Source: CAD feature listing. Evaluate the final solid. Frame: model axes, mm. A direction names the side the tool comes from. Give positions to 0.01 mm unless a question says otherwise; leave off trailing zeros. Loops run counter-clockwise (first coordinate to the right, second up) from the corner with the lowest first, then second, coordinate; pieces in that order, holes last.
from build123d import *

# Parameters (mm, degrees)
BOSS_EXTRUDE1_DEPTH            = 62
CONVERT_SOLID1_DEPTH           = 62
CONVERT_SOLID1_2_DEPTH         = 62
CUT_EXTRUDE2_DEPTH             = 79.552402891
SKETCH9_W                      = 18.8
SKETCH9_H                      = 20
CUT_EXTRUDE3_DEPTH             = 79.552402891
BOSS_EXTRUDE3_DEPTH            = 1.2
BOSS_EXTRUDE4_DEPTH            = 20
CUT_EXTRUDE4_DEPTH             = 20.58
CUT_EXTRUDE4_DIRECTION_2_REACH = 81.822
CHAMFER4_SIZE                  = 4
CHAMFER1_SIZE                  = 1.5
SKETCH7_R                      = 2.7686
CUT_EXTRUDE1_DEPTH             = 1.2


# Read off the part's stored shape, not the designer's step: Convert-Solid1
with BuildPart() as part:
    # Sketch2 → Boss-Extrude1 (new body)
    with BuildSketch(Plane(origin=(0, 0, 0), x_dir=(1, 0, 0), z_dir=(0, 1, 0))):
        Polygon((10, 0), (3, 0), (-3.915434451, 19), (-43.8, 19), (-43.8, 40), (10, 40), align=None)
    extrude(amount=BOSS_EXTRUDE1_DEPTH)

    # Convert-Solid1 outline → Convert-Solid1 (cut)
    with BuildSketch(Plane(origin=(0, 0, 0), x_dir=(1, 0, 0), z_dir=(0, 1, 0))):
        with BuildLine():
            ThreePointArc((4.680498092, 0), (3.303914645, 0.434035094), (2.425235802, 1.579151656))
            Line((2.425235802, 1.579151656), (3, 0))
            Line((3, 0), (4.680498092, 0))
        make_face()
        with BuildLine():
            Line((-43.8, 40), (-43.8, 20.2))
            Line((-43.8, 20.2), (-4.755683497, 20.2))
            ThreePointArc((-4.755683497, 20.2), (-3.37910005, 19.765964906), (-2.500421207, 18.620848344))
            Line((-2.500421207, 18.620848344), (3.552866947, 1.989575828))
            ThreePointArc((3.552866947, 1.989575828), (3.992206368, 1.417017547), (4.680498092, 1.2))
            Line((4.680498092, 1.2), (10, 1.2))
            Line((10, 1.2), (10, 40))
            Line((10, 40), (-43.8, 40))
        make_face()
    extrude(amount=CONVERT_SOLID1_DEPTH, mode=Mode.SUBTRACT)

    # Convert-Solid1 2 outline → Convert-Solid1 2 (add)
    with BuildSketch(Plane(origin=(0, 0, 0), x_dir=(1, 0, 0), z_dir=(0, 1, 0))):
        with BuildLine():
            ThreePointArc((-4.755683497, 19), (-4.067391773, 18.782982453), (-3.628052352, 18.210424172))
            Line((-3.628052352, 18.210424172), (-3.915434451, 19))
            Line((-3.915434451, 19), (-4.755683497, 19))
        make_face()
    extrude(amount=CONVERT_SOLID1_2_DEPTH)

    # Sketch8 → Cut-Extrude2 (cut, through all)
    with BuildSketch(Plane.XY):
        Polygon((-8.8, 35), (-10.3748, 34.347696482), (-10.3748, -34.347696482), (-8.8, -35), align=None)
        Polygon((-8.8, 35.5), (-10.3748, 36.152303518), (-10.3748, 75), (-8.8, 75), align=None)
        Polygon((-10.3748, -36.152303518), (-10.3748, -75), (-8.8, -75), (-8.8, -35.5), align=None)
    extrude(amount=-CUT_EXTRUDE2_DEPTH, mode=Mode.SUBTRACT)

    # Sketch9 → Cut-Extrude3 (cut, through all)
    with BuildSketch(Plane.XY):
        with Locations((0.6, 52)):
            Rectangle(SKETCH9_W, SKETCH9_H)
    extrude(amount=-CUT_EXTRUDE3_DEPTH, mode=Mode.SUBTRACT)

    # Sketch11 → Boss-Extrude3 (add)
    with BuildSketch(Plane.XY):
        Polygon((-3.1496, 43.5748), (4.680498092, 43.5748), (4.680498092, 42), (10, 42), (10, 62), (-10, 62), (-10, 50.4252), align=None)
    extrude(amount=-BOSS_EXTRUDE3_DEPTH)

    # Sketch12 → Boss-Extrude4 (add)
    with BuildSketch(Plane(origin=(0, 42, 0), x_dir=(1, 0, 0), z_dir=(0, 1, 0))):
        with BuildLine():
            Line((-3.628052352, 18.210424172), (0.305179296, 7.403959033))
            Line((0.305179296, 7.403959033), (1.432810441, 7.814383205))
            Line((1.432810441, 7.814383205), (-2.500421207, 18.620848344))
            ThreePointArc((-2.500421207, 18.620848344), (-3.37910005, 19.765964906), (-4.755683497, 20.2))
            Line((-4.755683497, 20.2), (-8.8, 20.2))
            Line((-8.8, 20.2), (-8.8, 19))
            Line((-8.8, 19), (-4.755683497, 19))
            ThreePointArc((-4.755683497, 19), (-4.067391773, 18.782982453), (-3.628052352, 18.210424172))
        make_face()
    extrude(amount=BOSS_EXTRUDE4_DEPTH)

    # Sketch13 → Cut-Extrude4 (cut)
    with BuildSketch(Plane(origin=(2.649066665, 0, -0.964181415), x_dir=(0.34202014332566943, 0, 0.9396926207859082), z_dir=(-0.9396926207859082, 0, 0.34202014332566943))):
        Polygon((-6.853068201, 42), (-11.853068201, 47), (-26.853068201, 47), (-26.853068201, 62), (-6.853068201, 62), align=None)
    extrude(amount=-CUT_EXTRUDE4_DEPTH, mode=Mode.SUBTRACT)

    # Cut-Extrude4 direction 2: up to this plane
    cut_extrude4_direction_2_end = Plane(origin=(-8.8, 35.5, -20.2), z_dir=(1, 0, 0))
    # Sketch13 → Cut-Extrude4 direction 2 (cut, up to the surface)
    with BuildSketch(Plane(origin=(2.649066665, 0, -0.964181415), x_dir=(0.34202014332566943, 0, 0.9396926207859082), z_dir=(-0.9396926207859082, 0, 0.34202014332566943)), mode=Mode.PRIVATE) as cut_extrude4_direction_2_sk1:
        Polygon((-6.853068201, 42), (-11.853068201, 47), (-26.853068201, 47), (-26.853068201, 62), (-6.853068201, 62), align=None)
    cut_extrude4_direction_2_tool1 = split(extrude(cut_extrude4_direction_2_sk1.sketch, amount=CUT_EXTRUDE4_DIRECTION_2_REACH, mode=Mode.PRIVATE), bisect_by=cut_extrude4_direction_2_end, keep=Keep.BOTH, mode=Mode.PRIVATE)
    add(cut_extrude4_direction_2_tool1.solids().sort_by_distance((-3.001015, 54.133333, -16.487654))[0], mode=Mode.SUBTRACT)

    # Chamfer4
    chamfer4_edges = [part.edges().sort_by_distance(p)[0] for p in [
        (10, 62, -0.6),
    ]]
    chamfer(chamfer4_edges, length=CHAMFER4_SIZE)

    # Chamfer1
    chamfer1_edges = [part.edges().sort_by_distance(p)[0] for p in [
        (-10, 62, -0.6),
        (-8.8, 47, -19.6),
        (-43.8, 62, -19.6),
        (-10.3748, 62, -19.6),
    ]]
    chamfer(chamfer1_edges, length=CHAMFER1_SIZE)

    # Mirror1: part across plane


with BuildPart() as part_1:
    add(part.part)
    add(part.part.mirror(Plane(origin=(10, 0, 0), x_dir=(0, 0, 1), z_dir=(0, 1, 0))))

    # Sketch7 → Cut-Extrude1 (cut)
    with BuildSketch(Plane.XY):
        with Locations((0, 52.5)):
            Circle(SKETCH7_R)
        with BuildLine():
            Line((-2.7686, -54), (-2.7686, -51))
            ThreePointArc((-2.7686, -51), (0, -48.2314), (2.7686, -51))
            Line((2.7686, -51), (2.7686, -54))
            ThreePointArc((2.7686, -54), (0, -56.7686), (-2.7686, -54))
        make_face()
    extrude(amount=-CUT_EXTRUDE1_DEPTH, mode=Mode.SUBTRACT)


solid = part_1.part
1) Cut plane B-B (y = 52.5). Return loops of the section in (x, z), and give its area (3 significant figures).
Checks:
outline: (-43.8, -20.2) - (-10.37, -20.2) - (-10.37, -19) - (-43.8, -19) - close; (-10, -1.2) - (-2.77, -1.2) - (-2.77, 0) - (-10, 0) - close; (2.77, -1.2) - (10, -1.2) - (10, 0) - (2.77, 0) - close
area: 57.5 mm2
2) Contact query for flat-ended pins moving along their axis: P1, Ø4, axis at y = 34.5, z = -14.5, coming from the -X side; P2, Ø3, axis at x = 1.5, y = 31, coming from the +Z side; P3, Ø1, axis at x = -16.5, y = -47, coming from the +Z side. Output: stop coordinate, or through.
Checks:
P1: stops at x = -3.01
P2: stops at z = -0.69
P3: stops at z = -19
3) Ray query, probe 1 along Y at (x, z) = (0, -0.35); probe 2 along Z at (x, y) = (-38, -44.5); probe 3 along Z at (x, y) = (7, 17.5). Return the intervals inside material, ascending.
Checks:
probe 1: y = -62 to -56.77, -48.23 to -43.57, 43.57 to 49.73, 55.27 to 62
probe 2: z = -20.2 to -19
probe 3: z = -1.2 to 0
4) Cut plane C-C (z = -11). Return loops of the section in (x, y), and give its area (3 significant figures).
Checks:
outline: (-1, -45.83) - (0.27, -45.39) - (0.27, 45.39) - (-1, 45.83) - close
area: 116 mm2
5) Cut plane A-A (y = -26.5). Return loops of the section in (x, z).
Checks:
outline: (-43.8, -20.2) - (-10.37, -20.2) - (-10.37, -19) - (-43.8, -19) - close; (-8.8, -20.2) - (-4.76, -20.2) arc R2.4 ccw to (-2.5, -18.62) - (3.55, -1.99) arc R1.2 cw to (4.68, -1.2) - (10, -1.2) - (10, 0) - (4.68, 0) arc R2.4 ccw to (2.43, -1.58) - (-3.63, -18.21) arc R1.2 cw to (-4.76, -19) - (-8.8, -19) - close
6) Reachability of faces 1 (the cylindrical face through (0.061, -56.768, -0.592)), 2 (the flat face through (-3, -47, -17)), 3 (the flat face through (-3, 47, -17)), 4 (the flat face through (-6.623, 47.048, -0.592)) from +Z, -Z, +X, -X, +Y, -Y: full face, straight path, thin tool, end or side. Return the list, or none.
Checks:
face 1: +Z, -Z
face 2: -Z, +X, -Y
face 3: -Z, +X, +Y
face 4: +Z, -X
7) Cut plane D-D (x = -19). Return loops of the section in (y, z).
Checks:
outline: (-62, -20.2) - (62, -20.2) - (62, -19) - (-62, -19) - close
8) Pull-direction query (Z, two-part tool) for faces 5 (the cylindrical face through (3.321, 0.588, -0.422)), 6 (the flat face through (-6.623, -47.048, -0.592)), 7 (the flat face through (0.02, 44.46, -9.92)), 8 (the flat face through (0.02, -44.46, -9.92)); classes: released by +Z, released by -Z, zero draft, split by the parting line, or undercut.
Checks:
face 5: released by +Z
face 6: zero draft
face 7: undercut
face 8: undercut
